Check sheet for the modelled part. Datum: model origin and axes. Units: mm. Face numbers are marked on the shaded views. Round coordinates to 2 decimals unless told otherwise and drop trailing zeros. Loops run counter-clockwise (first coordinate to the right, second up) from the corner with the lowest first, then second, coordinate; pieces in that order, holes last. Notation, with made-up numbers: (31, 46.25) - (73, 46.25) arc R6 ccw to (73, 56.25) - close; hole circle Ø9 at (-5, 7.25). An arc over 180 degrees is marked (long way). Put each result on its own line as item: value.
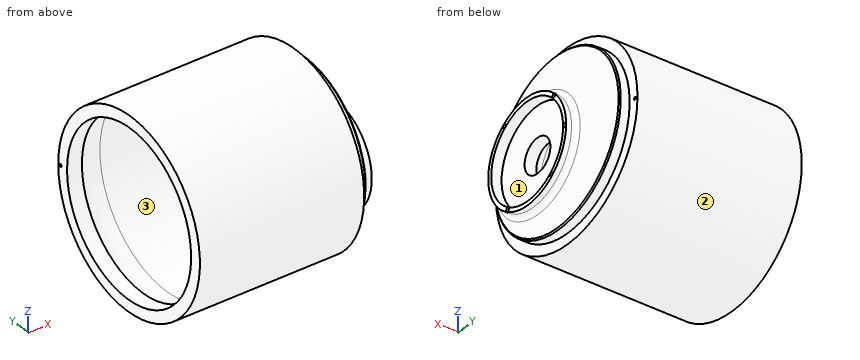
Autodesk Fusion 360 part; units mm, degrees
sketch "Sketch1" plane through (0, 0, 0) normal (0, 0, 1) x (1, 0, 0)
sketch "Sketch2" plane through (0, 0, 0) normal (0, 0, 1) x (1, 0, 0)
  line L0 (0, 0) -> (-4.064, 0)
  line L1 (-403.86, 200.025) -> (-367.284, 200.025)
  line L2 (-91.44, 219.075) -> (-308.5474, 219.075)
  line L3 (-403.86, 200.025) -> (-403.86, 228.346)
  line L4 (-403.86, 228.346) -> (-4.064, 228.346)
  line L5 (-4.064, 131.699) -> (-4.064, 0)
  arc A0 (-4.064, 131.699) -> (-91.44, 219.075) centre (-91.44, 131.699) ccw
  line L6 (-403.86, 228.346) -> (0, 228.346)
  line L7 (0, 228.346) -> (0, 219.075)
  line L8 (0, 219.075) -> (0, 0)
  arc A1 (-308.5474, 219.075) -> (-367.284, 200.025) centre (-318.7192, 150.3616) ccw
  dimension "d10" = 87.376
  dimension "d11" = 403.86
  dimension "d12" = 9.271
revolve "Revolve1" add sketch "Sketch2" angle 360 about axis through (1.75, 0, 0) along (1, 0, 0)
sketch "Sketch3" plane through (0, 0, 0) normal (1, 0, 0) x (0, 0, -1)
  circle A0 centre (0, 0) radius 228.346
  line L0 (0, 228.346) -> (0, 203.073)
  circle A1 centre (0, 0) radius 203.073
  dimension "d16" = 25.273
extrude "Extrude1" add sketch "Sketch3" along normal blind 24.892 contours A1
sketch "Sketch4" plane through (24.892, 0, 0) normal (1, 0, 0) x (0, 0, -1)
  circle A0 centre (0, 0) radius 203.073
  circle A1 centre (0, -61.341) radius 125.476
  circle A2 centre (0, -61.341) radius 115.8875
  dimension "d20" = 231.775
chamfer "Chamfer1" distance 3.048 angle 45 1 edges at (24.892, -73.4343, 189.3305)
extrude "Extrude2" add sketch "Sketch4" along normal blind 25.4 contours A1
fillet "Fillet1" radius 11.938 1 edges at (24.892, -15.9669, 116.9847)
sketch "Sketch5" plane through (24.892, 0, 0) normal (1, 0, 0) x (0, 0, -1)
  circle A0 centre (0, -61.341) radius 115.8875
  circle A1 centre (0, -61.341) radius 41.5925
  dimension "d25" = 83.185
extrude "Extrude3" cut sketch "Sketch5" against normal blind 889 contours A1
sketch "Sketch6" plane through (-403.86, 0, 0) normal (-1, 0, 0) x (0, 0, 1)
  circle A0 centre (0, 0) radius 200.025
  circle A1 centre (0, 0) radius 228.346
  line L0 (0, 228.346) -> (0, 220.726)
  circle A2 centre (0, 220.726) radius 3.2004
  dimension "d28" = 7.62
  dimension "d29" = 6.4008
extrude "Extrude4" cut sketch "Sketch6" against normal blind 8.128 contours A2
sketch "Sketch7" plane through (0, 0, 0) normal (1, 0, 0) x (0, 0, -1)
  circle A0 centre (0, 0) radius 203.073
  circle A1 centre (0, 0) radius 228.346
  line L0 (0, 228.346) -> (0, 220.218)
  circle A2 centre (0, 220.218) radius 3.2004
  dimension "d32" = 8.128
  dimension "d33" = 6.4008
extrude "Extrude5" cut sketch "Sketch7" against normal blind 8.128 contours A2
sketch "Sketch8" plane through (50.292, 0, 0) normal (1, 0, 0) x (0, 0, -1)
  circle A0 centre (0, -61.341) radius 115.8875
  circle A1 centre (0, -61.341) radius 125.476
  circle A2 centre (0.0718, 59.2759) radius 4.7625
  dimension "d36" = 9.525
hole "Hole1" at (50.292, 59.2759, -0.0718) direction (-1, 0, 0) diameter 9.144 depth 25.4 tip angle 180
hole "Hole2" at (50.292, 16.31, -92.4949) direction (-1, 0, 0) diameter 9.144 depth 25.4 tip angle 180
hole "Hole3" at (50.292, 23.8114, 85.7159) direction (-1, 0, 0) diameter 9.144 depth 25.4 tip angle 180
hole "Hole4" at (50.292, -135.0672, 95.7736) direction (-1, 0, 0) diameter 9.144 depth 25.4 tip angle 180
hole "Hole5" at (50.292, -124.6176, -102.8884) direction (-1, 0, 0) diameter 9.144 depth 25.4 tip angle 180
equation "d12 = ( ( 17.98 - 17.25 ) / 2 ) * 1 in"
equation "d16 = ( 1.99 / 2 ) * 1 in"
Item 1: Release check for a two-part mould opening along X. For the marked faces 1, 2 and 3 record: +X half, -X half, draft (parallel to the pull), parting line (faces both ways), or undercut.
Filled sheet:
face 1: +X half
face 2: draft
face 3: undercut
Item 2: Thickness scan on line 1 (Z direction, x = -203.5, y = 0) (3 decimals); line 2 (Z direction, x = -378.5, y = 2) (3 decimals); line 3 (Y direction, x = 11, z = 0). Record the ranges inside material, lowest first. Write a range as from..to.
Filled sheet:
line 1: -228.346..-219.075, 219.075..228.346
line 2: -228.337..-200.015, 200.015..228.337
line 3: -203.07..-102.93, -19.75..203.07
Item 3: Section check A-A on x = -179.5. Enter the section's corners in (y, z) (3 decimals), then the cut area to 3 significant figures.
Filled sheet:
outline: circle Ø456.692 at (0, 0); hole circle Ø438.15 at (0, 0)
area: 13,000 mm²
Item 4: Section check B-B on x = -72. Enter the section's corners in (y, z).
Filled sheet:
outline: circle Ø456.69 at (0, 0); hole circle Ø433.77 at (0, 0)
Item 5: Go/stop test with flat-tipped pins: pin 1 (7.5 mm diameter, centred on y = 16.31, z = -92.49, fed in from +X); pin 2 (10 mm diameter, centred on y = -65, z = 31.5, fed in from +X); pin 3 (5 mm diameter, centred on y = 221, z = -0.5, fed in from -X); pin 4 (1.5 mm diameter, centred on x = -125.5, z = 20.5, fed in from +Y). Record where each tip stops, or that it passes through.
Filled sheet:
pin 1: x = 24.89
pin 2: through
pin 3: x = -395.73
pin 4: y = 227.49
